Work out the finished part from the listing and answer in its coordinate system (mm). Round coordinates to 2 decimals unless told otherwise and drop trailing zeros. Order: outer loops, then holes, each group sorted by start corner. A loop starts at its lowest first (then second) coordinate and runs counter-clockwise, first axis right, second up. Notation, with made-up numbers: M -35.75,40 L -6.75,40 A6 ccw -6.75,50 Z; hole C -12.75,-12 d11. An arc over 180 degrees is marked long. Return JSON: item names as keys, results as strings.
from build123d import *

# Parameters (mm, degrees)
SKETCH1_W           = 155.2448
SKETCH1_H           = 117.1448
BOSS_EXTRUDE1_DEPTH = 2.54
SKETCH2_R           = 1.5875
SKETCH2_R_2         = 3.175
SKETCH2_R_3         = 4.7625
SKETCH2_R_4         = 1.5
SKETCH2_W           = 76.2
SKETCH2_H           = 26
CUT_EXTRUDE1_DEPTH  = 2.54


with BuildPart() as part:
    # Sketch1 → Boss-Extrude1 (new body)
    with BuildSketch(Plane(origin=(0, 0, 0), x_dir=(1, 0, 0), z_dir=(0, 1, 0))):
        with Locations((77.6224, 58.5724)):
            Rectangle(SKETCH1_W, SKETCH1_H)
    extrude(amount=BOSS_EXTRUDE1_DEPTH)

    # Sketch2 → Cut-Extrude1 (cut)
    with BuildSketch(Plane(origin=(0, 2.54, 0), x_dir=(1, 0, 0), z_dir=(0, 1, 0))):
        with Locations((31.097, 86.0978)):
            Circle(SKETCH2_R)
        with Locations((31.097, 31.0978)):
            Circle(SKETCH2_R)
        with Locations((124.097, 86.0978)):
            Circle(SKETCH2_R)
        with Locations((124.097, 31.0978)):
            Circle(SKETCH2_R)
        with Locations((12.047, 71.5978)):
            Circle(SKETCH2_R_2)
        with Locations((12.047, 46.1978)):
            Circle(SKETCH2_R_2)
        with Locations((12.047, 20.7978)):
            Circle(SKETCH2_R_3)
        with Locations((23.247, 20.7978)):
            Circle(SKETCH2_R_4)
        with Locations((77.597, 58.5978)):
            Rectangle(SKETCH2_W, SKETCH2_H)
    extrude(amount=-CUT_EXTRUDE1_DEPTH, mode=Mode.SUBTRACT)


solid = part.part
Item 1: Find section C-C (x = 11.5). Determine the outline of the cut face in (y, z).
Output:
{"outline": "M 0,-117.14 L 2.54,-117.14 L 2.54,-74.73 L 0,-74.73 Z; M 0,-68.47 L 2.54,-68.47 L 2.54,-49.33 L 0,-49.33 Z; M 0,-43.07 L 2.54,-43.07 L 2.54,-25.53 L 0,-25.53 Z; M 0,-16.07 L 2.54,-16.07 L 2.54,0 L 0,0 Z"}
Item 2: The mould has two halves that part along X. Classify faces 1 (the flat face through (77, 2.54, -72)), 2 (the cylindrical face through (124.95, 1.288, -87.436)), 3 (the cylindrical face through (11.36, 1.29, -43.1)): pulls with the +X half, pulls with the -X half, needs draft (parallel to the pull), parting line crosses it, or undercut.
Output:
{"face 1": "needs draft", "face 2": "undercut", "face 3": "undercut"}
Item 3: Find section D-D (y = 1.9). State how many separate pieces and enclosed holes the cut face has, plus the area to 3 significant figures.
Output:
{"separate pieces": "1", "enclosed holes": "9", "area": "16,000 mm^2"}
Item 4: Consider line 1 along Z through (x, y) = (48.5, 2.3); line 2 along Z through (x, y) = (31, 0.5); line 3 along X through (y, z) = (1.6, -63.5). Determine where each line is inside the solid, lowest interval first. Write a range as [from, to].
Output:
{"line 1": "z = [-117.14, -71.6], [-45.6, 0]", "line 2": "z = [-117.14, -87.68], [-84.51, -32.68], [-29.51, 0]", "line 3": "x = [0, 39.5], [115.7, 155.24]"}
Item 5: Find section B-B (z = -54.5). Determine the outline of the cut face in (x, y).
Output:
{"outline": "M 0,0 L 39.5,0 L 39.5,2.54 L 0,2.54 Z; M 115.7,0 L 155.24,0 L 155.24,2.54 L 115.7,2.54 Z"}
Item 6: Find section A-A (x = 60). Determine the outline of the cut face in (y, z).
Output:
{"outline": "M 0,-117.14 L 2.54,-117.14 L 2.54,-71.6 L 0,-71.6 Z; M 0,-45.6 L 2.54,-45.6 L 2.54,0 L 0,0 Z"}
